Autodesk Inventor part; units mm, degrees
ref_plane "YZ Plane" through (0, 0, 0) normal (1, 0, 0) x (0, 1, 0)
ref_plane "XZ Plane" through (0, 0, 0) normal (0, 1, 0) x (-1, 0, 0)
ref_plane "XY Plane" through (0, 0, 0) normal (0, 0, 1) x (1, 0, 0)
sketch "Sketch1" plane through (0, 0, 0) normal (0, 0, 1) x (1, 0, 0)
  line L0 (-67.5, -15) -> (67.5, -15)
  line L1 (67.5, -15) -> (67.5, 15)
  line L2 (67.5, 15) -> (-67.5, 15)
  line L3 (-67.5, 15) -> (-67.5, -15)
  line L4 (-67.5, -15) -> (67.5, 15) construction
  line L5 (67.5, -15) -> (-67.5, 15) construction
  line L6 (-20.5, -8.8) -> (20.5, -8.8)
  line L7 (20.5, -8.8) -> (20.5, -12)
  line L8 (20.5, -12) -> (-20.5, -12)
  line L9 (-20.5, -12) -> (-20.5, -8.8)
  line L10 (-20.5, -8.8) -> (20.5, -12) construction
  line L11 (20.5, -8.8) -> (-20.5, -12) construction
  point P0 (0, 0)
  point P1 (0, -10.4)
  point P2 (0, -8.8)
  dimension "d0" = 135
  dimension "d1" = 30
  dimension "d5" = 41
  dimension "d6" = 3
  dimension "d7" = 3.2
extrude "Plate1" add sketch "Sketch1" along normal mid plane 3
equation "\"d4\" = Thickness"
equation "\"BendRadius\" = Thickness"
equation "\"BendReliefWidth\" = Thickness"
equation "\"BendReliefDepth\" = 0.5 * Thickness"
equation "\"CornerReliefSize\" = 4 * Thickness"
equation "\"MinimumRemnant\" = 2 * Thickness"
equation "\"TransitionRadius\" = BendRadius"
equation "\"JacobiRadiusSize\" = BendRadius"
equation "\"GapSize\" = Thickness"
properties part number "Path Side Wall"
Verification items for the finished model (mm, model axes). A direction names the side the tool comes from. Coordinates: 2 decimals unless noted, no trailing zeros. Order: outer loops, then holes, each group sorted by start corner. A loop starts at its lowest first (then second) coordinate and runs counter-clockwise, first axis right, second up. Notation, with made-up numbers: M 50.5,23.5 L 105.5,23.5 A29 cw 105.5,58.5 Z; hole C 43,48 d3. An arc over 180 degrees is marked long. One line per item, written item: value. Start each with the question number.
Item 1: Sectioned sample at A-A (x = -7). Enter the section's corners in (y, z), then the cut area to 3 significant figures.
Item 2: Mould release check, pull along X, two halves, no side actions. Record for faces 1 (the flat face through (0, -8.8, 0)), 2 (the flat face through (67.5, 0, 0)), 3 (the flat face through (-1, 0, 1.5)): released by +X, released by -X, zero draft, split by the parting line, or undercut.
Item 3: Scan lines: probe 1 along X at (y, z) = (-10.5, -0.9); probe 2 along Y at (x, z) = (16, 0.8). Record each from-to range of solid material in increasing order.
Item 4: Access from +Z, -Z, +X, -X, +Y, -Y to the whole of each face (thin tool, end or side, straight path). Record for faces 4 (the flat face through (1, 15, 0)), 5 (the flat face through (-20.5, -10, 0)).
Item 5: Sectioned sample at B-B (z = 0). Enter the section's corners in (x, y), then the cut area to 3 significant figures.
Item 6: Gauge pin test, flat end, axial feed: pin 1 (12 mm diameter, centred on x = -6.5, y = -9, fed in from -Z). Record the tip position at first contact, or that the pin passes through.
Conclusion:
1. outline: M -15,-1.5 L -12,-1.5 L -12,1.5 L -15,1.5 Z; M -8.8,-1.5 L 15,-1.5 L 15,1.5 L -8.8,1.5 Z
1. area: 80.4 mm^2
2. face 1: undercut
2. face 2: released by +X
2. face 3: zero draft
3. probe 1: x = -67.5 to -20.5, 20.5 to 67.5
3. probe 2: y = -15 to -12, -8.8 to 15
4. face 4: +Z, -Z, +X, -X, +Y
4. face 5: +Z, -Z
5. outline: M -67.5,-15 L 67.5,-15 L 67.5,15 L -67.5,15 Z; hole M -20.5,-12 L 20.5,-12 L 20.5,-8.8 L -20.5,-8.8 Z
5. area: 3,920 mm^2
6. pin 1: stops at z = -1.5
